Design review of the part built by this model. Coordinates are the model's own, in mm. A direction names the side the tool comes from. Round coordinates to 2 decimals unless told otherwise and drop trailing zeros. Write each loop counter-clockwise with the first axis right and the second up, starting at its lowest first coordinate (ties: lowest second). Pieces come first, ordered by that corner, then holes. Notation, with made-up numbers: M 74,70 L 111,70 A5 ccw 111,76 Z; hole C 78,65.25 d7. An arc over 180 degrees is marked long. Use CSV: the item, a comma, the result in double quotes.
from build123d import *

# Parameters (mm, degrees)
EXTRUSION1_DEPTH = 13
ESQUISSE2_R      = 2
EXTRUSION2_DEPTH = 3


with BuildPart() as part:
    # Esquisse1 → Extrusion1 (new body)
    with BuildSketch(Plane.XY):
        Polygon((-30.903636364, 29.709316239), (-30.903636364, 24.450320542), (-35.903636364, 24.450320542), (-35.903636364, 22.450320542), (-30.903636364, 22.450320542), (-30.903636364, 6.709316239), (-8.403636364, 6.709316239), (-8.403636364, 22.450320542), (-3.403636364, 22.450320542), (-3.403636364, 24.450320542), (-8.403636364, 24.450320542), (-8.403636364, 29.709316239), align=None)
    extrude(amount=EXTRUSION1_DEPTH)

    # Esquisse2 → Extrusion2 (add)
    with BuildSketch(Plane(origin=(0, 29.709316239, 0), x_dir=(1, 0, 0), z_dir=(0, 1, 0))):
        with Locations(Location((-14.903636364, -6.5, 0), (0, 0, 90))):
            Circle(ESQUISSE2_R)
    extrude(amount=EXTRUSION2_DEPTH)


solid = part.part
1) Add section A-A on z = 10. Write out the cut boundary in (x, y).
Answers:
outline,"M -35.9,22.45 L -30.9,22.45 L -30.9,6.71 L -8.4,6.71 L -8.4,22.45 L -3.4,22.45 L -3.4,24.45 L -8.4,24.45 L -8.4,29.71 L -30.9,29.71 L -30.9,24.45 L -35.9,24.45 Z"
2) Add section D-D on y = 14. Write out the cut boundary in (x, z).
Answers:
outline,"M -30.9,0 L -8.4,0 L -8.4,13 L -30.9,13 Z"
3) Add section C-C on z = 6.5. Write out the cut boundary in (x, y).
Answers:
outline,"M -35.9,22.45 L -30.9,22.45 L -30.9,6.71 L -8.4,6.71 L -8.4,22.45 L -3.4,22.45 L -3.4,24.45 L -8.4,24.45 L -8.4,29.71 L -12.9,29.71 L -12.9,32.71 L -16.9,32.71 L -16.9,29.71 L -30.9,29.71 L -30.9,24.45 L -35.9,24.45 Z"
4) For pin 1 Ø2.5 at (x, z) = (-6.5, 5) entering from +Y; pin 2 Ø5.5 at (x, z) = (-34, 7) entering from -Y; pin 3 Ø5 at (x, z) = (-21.5, 11) entering from +Y, all flat-tipped, find the tip position at first contact; note any pin that passes through.
Answers:
pin 1,"y = 24.45"
pin 2,"y = 22.45"
pin 3,"y = 29.71"
5) Add section B-B on x = -6. Write out the cut boundary in (y, z).
Answers:
outline,"M 22.45,0 L 24.45,0 L 24.45,13 L 22.45,13 Z"
6) Machinability: for faces 1 (the face through (-8.404, 14, 6)), 2 (the face through (-8.404, 27, 6)), 3 (the face through (-30.904, 27, 6)), which of the approach directions +Z, -Z, +X, -X, +Y, -Y give a long, thin tool a straight path to every point of the face, cutting with its end or side? Answer none if there is none.
Answers:
face 1,"+Z, -Z, +X, -Y"
face 2,"+Z, -Z, +X, +Y"
face 3,"+Z, -Z, -X, +Y"
7) Wall thickness on line 1 along Y through (x, z) = (-6, 4.75); line 2 along Y through (x, z) = (-10.5, 7); line 3 along X through (y, z) = (9, 0.75): over which ranges is each line inside the solid? List them lowest first. Write a range as [from, to].
Answers:
line 1,"[22.45, 24.45]"
line 2,"[6.71, 29.71]"
line 3,"[-30.9, -8.4]"
